Build history of the part. All positions in model axes, mm. Face numbers are marked on the shaded views. A direction names the side the tool comes from. Round coordinates to 2 decimals unless told otherwise and drop trailing zeros. Write each loop counter-clockwise with the first axis right and the second up, starting at its lowest first coordinate (ties: lowest second). Pieces come first, ordered by that corner, then holes.
1) Saw through at B-B (z = 8). Write the cut outline in (x, y).
2) Which spindle directions (+Z, -Z, +X, -X, +Y, -Y) get a long thin tool onto all of the face, cutting with end or side? Do the marked faces 1 and 2. Say none if no direction does.
3) Saw through at C-C (y = 9). Write the cut outline in (x, z).
4) Saw through at D-D (z = 4). Write the cut outline in (x, y), plus the area to 3 significant figures.
5) Saw through at A-A (x = 0). Write the cut outline in (y, z).
6) Flat gauge pins, fed straight in: pin 1 (10 mm diameter, centred on y = 22.5, z = 4, fed in from +X); pin 2 (8 mm diameter, centred on y = -3, z = -11.5, fed in from -X); pin 3 (1.5 mm diameter, centred on x = -3, y = -7.5, fed in from -Z). Where does each tip first touch, or does it go through?
7) Wall check: probe 1 along Y at (x, z) = (-9, -2); probe 2 along X at (y, z) = (-1, 4); probe 3 along Y at (x, z) = (5.5, -15). Give the ranges that are in metal, low to high.
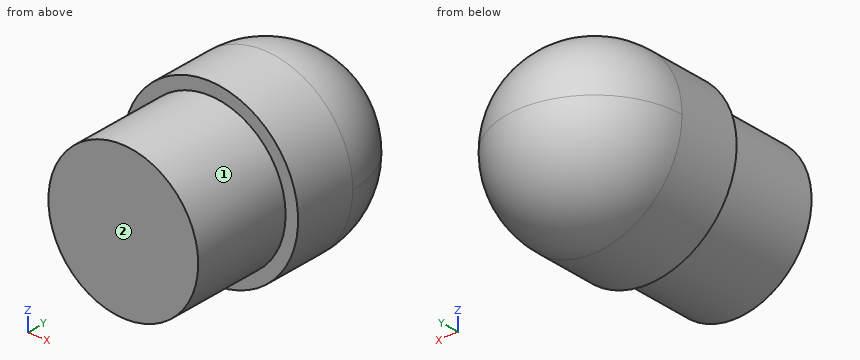
from build123d import *

# Parameters (mm, degrees)
F0_R     = 15
F1_DEPTH = 20
F2_R     = 17.5
F2_R_2   = 15
F3_DEPTH = 12.5


with BuildPart() as f1:
    # F0 (on Front) → F1 (new body)
    with BuildSketch(Plane.XZ):
        Circle(F0_R)
    extrude(amount=F1_DEPTH)

    # F2 (on face) → F3 (join)
    with BuildSketch(Plane(origin=(0, 0, 0), x_dir=(-1, 0, 0), z_dir=(0, 1, 0))):
        Circle(F2_R)
        Circle(F2_R_2, mode=Mode.SUBTRACT)
        Circle(F2_R_2)
    extrude(amount=F3_DEPTH)

    # F4 (on face) → F5 (revolve)
    with BuildSketch(Plane(origin=(0, 12.5, 0), x_dir=(-1, 0, 0), z_dir=(0, 1, 0))):
        with BuildLine():
            ThreePointArc((17.5, 0), (12.3743686708, 12.3743686708), (0, 17.5))
            Line((0, 17.5), (0, -17.5))
            ThreePointArc((0, -17.5), (12.3743686708, -12.3743686708), (17.5, 0))
        make_face()
    revolve(axis=Axis((0, 12.5, 0), (0, 0, -1)))


solid = f1.part
Evaluation:
1. outline: (-15.56, 0) - (-12.69, 0) - (-12.69, -20) - (12.69, -20) - (12.69, 0) - (15.56, 0) - (15.56, 12.5) arc R15.56 ccw to (-15.56, 12.5) - close
2. face 1: -Y
2. face 2: +Z, -Z, +X, -X, -Y
3. outline: circle Ø35 at (0, 0)
4. outline: (-17.04, 0) - (-14.46, 0) - (-14.46, -20) - (14.46, -20) - (14.46, 0) - (17.04, 0) - (17.04, 12.5) arc R17.04 ccw to (-17.04, 12.5) - close
4. area: 1,460 mm2
5. outline: (-20, -15) - (0, -15) - (0, -17.5) - (12.5, -17.5) arc R17.5 ccw to (12.5, 17.5) - (0, 17.5) - (0, 15) - (-20, 15) - close
6. pin 1: stops at x = 16.52
6. pin 2: stops at x = -15.09
6. pin 3: stops at z = -14.83
7. probe 1: y = -20 to 27.37
7. probe 2: x = -14.46 to 14.46
7. probe 3: y = 0 to 19.64
